Build history of the part. All positions in model axes, mm. A direction names the side the tool comes from. Coordinates: 2 decimals unless noted, no trailing zeros. Loops run counter-clockwise (first coordinate to the right, second up) from the corner with the lowest first, then second, coordinate; pieces in that order, holes last.
(1) Wall check: L1, parallel to X at y = -6, z = 1.45; L2, parallel to X at y = -22.5, z = 2.2; L3, parallel to X at y = -65, z = 0.3 (3 decimals). Give the ranges that are in metal, low to high.
(2) Slice it at C-C (x = -17). Give the cut face in (y, z).
(3) Slice it at B-B (y = 72). Give the cut face in (x, z), and give its area (3 significant figures).
(4) Tool access for faces 1 (the face through (4.403, -73.145, 0.986)), 2 (the face through (-10.02, -39.52, 1.52)): list every direction of +Z, -Z, +X, -X, +Y, -Y with a clear straight run to the whole face (end or side of a thin tool).
(5) Slice it at A-A (y = -84). Give the cut face in (x, z), and give its area (3 significant figures).
(6) Two-plate mould, pull along X, no slides. Class faces 3 (the face through (0.521, 28.966, 1.479)), 4 (the face through (16.29, 74.72, 1.48)): pulls with the +X half, pulls with the -X half, needs draft (parallel to the pull), parting line crosses it, or undercut.
(7) Flat gauge pins, fed straight in: P1, Ø2.5, axis at x = 0, y = 33, coming from the -Z side; P2, Ø0.9, axis at y = -53, z = 1.5, coming from the -X side. Where does each tip first touch, or does it go through?
(8) Slice it at D-D (z = 1.2). Give the number of separate pieces and of enclosed holes in the cut face, and give its area (3 significant figures).
from build123d import *

# Parameters (mm, degrees)
EXTRUDE_1_DEPTH              = 3
CUT_EXTRUDE_1_REACH          = 104.025
SKETCH_2_W                   = 5
SKETCH_2_H                   = 10
HOLE_WIZARD_M2_1_D           = 2.4
HOLE_WIZARD_M2_1_CBORE_D     = 4.4
HOLE_WIZARD_M2_1_CBORE_DEPTH = 2
CUT_EXTRUDE_2_REACH          = 104.025
SKETCH_5_R                   = 4
HOLE_WIZARD_M2_2_D           = 2.4
HOLE_WIZARD_M2_2_CBORE_D     = 4.4
HOLE_WIZARD_M2_2_CBORE_DEPTH = 2
HOLE_WIZARD_M2_3_D           = 2.4
HOLE_WIZARD_M2_3_CBORE_D     = 4.4
HOLE_WIZARD_M2_3_CBORE_DEPTH = 2
CUT_EXTRUDE_3_DEPTH          = 3
HOLE_WIZARD_M2_5_D           = 2.4
HOLE_WIZARD_M2_5_CBORE_D     = 4.4
HOLE_WIZARD_M2_5_CBORE_DEPTH = 2


with BuildPart() as part:
    # 草图1 → 凸台-拉伸1 (new body)
    with BuildSketch(Plane.XY):
        Polygon((20, 5), (20, 45), (19.258297735, 54.944681764), (13.241702265, 95.055318236), (7.5, 100), (-7.5, 100), (-13.241702265, 95.055318236), (-19.258297735, 54.944681764), (-20, 45), (-20, 5), (-19.379826327, -4.961389384), (-7.748069469, -98.015444247), (-5.5, -100), (5.5, -100), (7.748069469, -98.015444247), (19.379826327, -4.961389384), align=None)
    extrude(amount=EXTRUDE_1_DEPTH)

    # 草图2 → 切除-拉伸1 (cut, up to next)
    with BuildSketch(Plane.XY.offset(3), mode=Mode.PRIVATE) as cut_extrude_1_sk1:
        Polygon((10, -5), (-10, -5), (0, -22.320508076), align=None)
    cut_extrude_1_tool1 = extrude(cut_extrude_1_sk1.sketch, amount=-CUT_EXTRUDE_1_REACH, mode=Mode.PRIVATE) & part.part
    # 草图2 → 切除-拉伸1 (cut, up to next)
    with BuildSketch(Plane.XY.offset(3), mode=Mode.PRIVATE) as cut_extrude_1_sk2:
        Polygon((6.211088907, -70), (13.938881842, -8.177656525), (2.5, -27.990381057), (2.5, -70), align=None)
    cut_extrude_1_tool2 = extrude(cut_extrude_1_sk2.sketch, amount=-CUT_EXTRUDE_1_REACH, mode=Mode.PRIVATE) & part.part
    # 草图2 → 切除-拉伸1 (cut, up to next)
    with BuildSketch(Plane.XY.offset(3), mode=Mode.PRIVATE) as cut_extrude_1_sk3:
        Polygon((-13.938881842, -8.177656525), (-2.5, -27.990381057), (-2.5, -70), (-6.211088907, -70), align=None)
    cut_extrude_1_tool3 = extrude(cut_extrude_1_sk3.sketch, amount=-CUT_EXTRUDE_1_REACH, mode=Mode.PRIVATE) & part.part
    # 草图2 → 切除-拉伸1 (cut, up to next)
    with BuildSketch(Plane.XY.offset(3), mode=Mode.PRIVATE) as cut_extrude_1_sk4:
        with Locations((0, -85)):
            Rectangle(SKETCH_2_W, SKETCH_2_H)
    cut_extrude_1_tool4 = extrude(cut_extrude_1_sk4.sketch, amount=-CUT_EXTRUDE_1_REACH, mode=Mode.PRIVATE) & part.part
    add(cut_extrude_1_tool1.solids().sort_by_distance((0, -10.773503, 3))[0], mode=Mode.SUBTRACT)
    add(cut_extrude_1_tool2.solids().sort_by_distance((6.712708, -39.914502, 3))[0], mode=Mode.SUBTRACT)
    add(cut_extrude_1_tool3.solids().sort_by_distance((-6.712708, -39.914502, 3))[0], mode=Mode.SUBTRACT)
    add(cut_extrude_1_tool4.solids().sort_by_distance((0, -85, 3))[0], mode=Mode.SUBTRACT)

    # M2 凹头盖螺钉的柱形沉头孔1 (through all)
    with Locations(Plane(origin=(5.586088907, -75, 0), x_dir=(-1, 0, 0), z_dir=(0, 0, -1))):
        with Locations((0, 0), (11.172177814, 0)):
            CounterBoreHole(HOLE_WIZARD_M2_1_D / 2, HOLE_WIZARD_M2_1_CBORE_D / 2, HOLE_WIZARD_M2_1_CBORE_DEPTH)

    # 草图5 → 切除-拉伸2 (cut, up to next)
    with BuildSketch(Plane(origin=(0, 0, 0), x_dir=(-1, 0, 0), z_dir=(0, 0, -1)), mode=Mode.PRIVATE) as cut_extrude_2_sk1:
        with Locations((0, 25)):
            Circle(SKETCH_5_R)
    cut_extrude_2_tool1 = extrude(cut_extrude_2_sk1.sketch, amount=-CUT_EXTRUDE_2_REACH, mode=Mode.PRIVATE) & part.part
    add(cut_extrude_2_tool1.solids().sort_by_distance((0, 25, 0))[0], mode=Mode.SUBTRACT)

    # M2 凹头盖螺钉的柱形沉头孔2 (through all)
    with Locations(Plane(origin=(8, 25, 0), x_dir=(-1, 0, 0), z_dir=(0, 0, -1))):
        with Locations((0, 0), (8, 8), (16, 0), (8, -8)):
            CounterBoreHole(HOLE_WIZARD_M2_2_D / 2, HOLE_WIZARD_M2_2_CBORE_D / 2, HOLE_WIZARD_M2_2_CBORE_DEPTH)

    # M2 凹头盖螺钉的柱形沉头孔3 (through all)
    with Locations(Plane(origin=(12.880020708, -5.011657807, 0), x_dir=(-1, 0, 0), z_dir=(0, 0, -1))):
        with Locations((0, 0), (25.760041416, 0)):
            CounterBoreHole(HOLE_WIZARD_M2_3_D / 2, HOLE_WIZARD_M2_3_CBORE_D / 2, HOLE_WIZARD_M2_3_CBORE_DEPTH)

    # 草图10 → 切除-拉伸3 (cut)
    with BuildSketch(Plane(origin=(0, 0, 0), x_dir=(-1, 0, 0), z_dir=(0, 0, -1))):
        Polygon((-14.016935065, 56.180852205), (-10.679274874, 78.431920145), (-8.411945476, 80.068406675), (-4.470648492, 79.385634325), (-2.5, 77.04424815), (-2.5, 56.2029795), (-4.5, 54.2029795), (-12.313615971, 54.2029795), align=None)
        Polygon((-9.344020618, 87.333615184), (-8.2970205, 94.313615971), (0, 94.313615971), (8.2970205, 94.313615971), (9.344020618, 87.333615184), (7.670053032, 85.014356303), (0, 83.685631227), (-7.670053032, 85.014356303), align=None)
        Polygon((4.5, 54.2029795), (12.313615971, 54.2029795), (14.016935065, 56.180852205), (10.679274874, 78.431920145), (8.411945476, 80.068406675), (4.470648492, 79.385634325), (2.5, 77.04424815), (2.5, 56.2029795), align=None)
    extrude(amount=-CUT_EXTRUDE_3_DEPTH, mode=Mode.SUBTRACT)

    # M2 凹头盖螺钉的柱形沉头孔5 (through all)
    with Locations(Plane(origin=(0, 79.840052868, 0), x_dir=(-1, 0, 0), z_dir=(0, 0, -1))):
        with Locations((0, 0)):
            CounterBoreHole(HOLE_WIZARD_M2_5_D / 2, HOLE_WIZARD_M2_5_CBORE_D / 2, HOLE_WIZARD_M2_5_CBORE_DEPTH)


solid = part.part
Response values:
1. L1: x = -19.25 to -14.85, -10.91 to -9.42, 9.42 to 10.91, 14.85 to 19.25
1. L2: x = -17.19 to -12.15, -5.67 to 5.67, 12.15 to 17.19
1. L3: x = -11.875 to -6.836, -2.5 to 2.5, 6.836 to 11.875
2. outline: (-24, 0) - (70, 0) - (70, 3) - (-24, 3) - close
3. outline: (-16.7, 0) - (-11.64, 0) - (-11.64, 3) - (-16.7, 3) - close; (-2.5, 0) - (2.5, 0) - (2.5, 3) - (-2.5, 3) - close; (11.64, 0) - (16.7, 0) - (16.7, 3) - (11.64, 3) - close
3. area: 45.3 mm2
4. face 1: -Z
4. face 2: +Z, -Z
5. outline: (-9.5, 0) - (-2.5, 0) - (-2.5, 3) - (-9.5, 3) - close; (2.5, 0) - (9.5, 0) - (9.5, 3) - (2.5, 3) - close
5. area: 42.0 mm2
6. face 3: undercut
6. face 4: pulls with the +X half
7. P1: stops at z = 2
7. P2: stops at x = -13.43
8. separate pieces: 1
8. enclosed holes: 17
8. area: 4,560 mm2
